Design review of the part built by this model. Coordinates are the model's own, in mm. A direction names the side the tool comes from. Coordinates: 2 decimals unless noted, no trailing zeros. Write each loop counter-clockwise with the first axis right and the second up, starting at its lowest first coordinate (ties: lowest second). Pieces come first, ordered by that corner, then holes. Notation, with made-up numbers: (82, -2.5) - (113, -2.5) arc R8 ccw to (113, 2.5) - close; hole circle Ø2 at (79.5, 23.25). An arc over 180 degrees is marked (long way). One line per item, written item: value.
Autodesk Inventor part; units mm, degrees
ref_plane "YZ Plane" through (0, 0, 0) normal (1, 0, 0) x (0, 1, 0)
ref_plane "XZ Plane" through (0, 0, 0) normal (0, 1, 0) x (-1, 0, 0)
ref_plane "XY Plane" through (0, 0, 0) normal (0, 0, 1) x (1, 0, 0)
sketch "Sketch1" plane through (0, 0, 0) normal (0, 0, 1) x (1, 0, 0)
  line L0 (19.05, -4) -> (-19.05, -4)
  line L1 (-19.05, -4) -> (-19.05, 4)
  line L2 (-19.05, 4) -> (19.05, 4)
  line L3 (19.05, 4) -> (19.05, -4)
  line L4 (19.05, -4) -> (-19.05, 4) construction
  line L5 (-19.05, -4) -> (19.05, 4) construction
  circle A0 centre (11.05, 0) radius 2.25
  circle A1 centre (3.05, 0) radius 2.25
  circle A2 centre (-4.95, 0) radius 2.25
  circle A3 centre (-12.95, 0) radius 2.25
  line L6 (-19.05, 4) -> (-25.4, 4)
  line L7 (-25.4, 4) -> (-25.4, -34.1)
  line L8 (-25.4, -34.1) -> (-19.05, -34.1)
  line L9 (-19.05, -34.1) -> (-19.05, 4)
  line L10 (-25.4, -34.1) -> (-12.6924, -34.1) construction
  line L11 (-25.4, -34.1) -> (-6.35, -34.1)
  line L12 (-6.35, -34.1) -> (-6.35, -27.75)
  line L13 (-6.35, -27.75) -> (-25.4, -27.75)
  line L14 (-25.4, -27.75) -> (-25.4, -34.1)
  line L15 (-6.35, -34.1) -> (-17.257, -23.193)
  point P0 (0, 0)
  point P1 (-19.05, -27.75)
  point P2 (-12.7, -27.75)
  point P3 (-19.05, -27.75)
  dimension "d0" = 38.1
  dimension "d1" = 8
  dimension "d2" = 4.5
  dimension "d3" = 8
  dimension "d4" = 4.5
  dimension "d5" = 8
  dimension "d6" = 4.5
  dimension "d7" = 8
  dimension "d8" = 4.5
  dimension "d9" = 8
  dimension "d10" = 4
  dimension "d11" = 4
  dimension "d12" = 4
  dimension "d13" = 4
  dimension "d16" = 6.35
  dimension "d17" = 38.1
  dimension "d20" = 19.05
  dimension "d21" = 6.35
  dimension "d22" = 45
extrude "Extrusion1" add sketch "Sketch1" along normal blind 6.35 contours L0 L1 L2 L3 | L9 L13 L7 L6 L1 | L13 L15 L11 L9 | L9 L8 L7 L13
fillet "Fillet1" radius 3.175 5 edges at (-19.05, -27.75, 3.175) (-19.05, -4, 3.175) (-25.4, 4, 3.175) (19.05, 4, 3.175) (19.05, -4, 3.175)
fillet "Fillet2" radius 3.175 2 edges at (-12.7, -27.75, 3.175) (-25.4, -34.1, 3.175)
properties part number "CS_Latch_Hooks"
1. For faces 1 (the face through (-3, 4, 3)), 2 (the face through (-15, -27.75, 3)), list the 3-axis set-ups (+Z, -Z, +X, -X, +Y, -Y) from which the entire face can be reached by the end or side of a thin tool; tool diameter is ignored.
Answer block:
face 1: +Z, -Z, +X, -X, +Y
face 2: +Z, -Z, +X
2. Consider section B-B, the plane z = 1. Write out the cut boundary in (x, y) (3 decimals).
Answer block:
outline: (-25.4, -30.925) arc R3.175 ccw to (-22.225, -34.1) - (-6.35, -34.1) - (-11.77, -28.68) arc R3.175 ccw to (-14.015, -27.75) - (-15.875, -27.75) arc R3.175 cw to (-19.05, -24.575) - (-19.05, -7.175) arc R3.175 cw to (-15.875, -4) - (15.875, -4) arc R3.175 ccw to (19.05, -0.825) - (19.05, 0.825) arc R3.175 ccw to (15.875, 4) - (-22.225, 4) arc R3.175 ccw to (-25.4, 0.825) - close; hole circle Ø4.5 at (-12.95, 0); hole circle Ø4.5 at (-4.95, 0); hole circle Ø4.5 at (3.05, 0); hole circle Ø4.5 at (11.05, 0)
3. Mouldability with a two-part tool opening along Y and no side actions: class faces 3 (the face through (-9.9, -3.7, 6.35)), 4 (the face through (18.14, 3.05, 3.22)), 5 (the face through (-7.198, -0.099, 3.131)) as released by +Y, released by -Y, zero draft, split by the parting line, or undercut.
Answer block:
face 3: zero draft
face 4: released by +Y
face 5: undercut
4. Consider section C-C, the plane x = 2. Write out the cut boundary in (y, z), then the cut area to 3 significant figures.
Answer block:
outline: (-4, 0) - (-1.99, 0) - (-1.99, 6.35) - (-4, 6.35) - close; (1.99, 0) - (4, 0) - (4, 6.35) - (1.99, 6.35) - close
area: 25.5 mm^2
5. Wall thickness on line 1 along Y through (x, z) = (-4.95, 2); line 2 along Y through (x, z) = (-12.95, 3); line 3 along Y through (x, z) = (1.5, 1.5): over which ranges is each line inside the solid? List them lowest first.
Answer block:
line 1: y = -4 to -2.25, 2.25 to 4
line 2: y = -34.1 to -27.93, -4 to -2.25, 2.25 to 4
line 3: y = -4 to -1.63, 1.63 to 4
6. Insertion check: pin 1 Ø2.5 at (x, y) = (-4.95, 0) entering from -Z; pin 2 Ø1.5 at (x, z) = (5.5, 1.5) entering from -Y. Each pin has a flat end and moves straight along its axis. Give the tip position at first contact, or say it passes through.
Answer block:
pin 1: passes through
pin 2: stops at y = -4
7. Consider section A-A, the plane y = 0. Write out the cut boundary in (x, z).
Answer block:
outline: (-25.4, 0) - (-15.2, 0) - (-15.2, 6.35) - (-25.4, 6.35) - close; (-10.7, 0) - (-7.2, 0) - (-7.2, 6.35) - (-10.7, 6.35) - close; (-2.7, 0) - (0.8, 0) - (0.8, 6.35) - (-2.7, 6.35) - close; (5.3, 0) - (8.8, 0) - (8.8, 6.35) - (5.3, 6.35) - close; (13.3, 0) - (19.05, 0) - (19.05, 6.35) - (13.3, 6.35) - close
8. Consider section D-D, the plane x = -13. Write out the cut boundary in (y, z).
Answer block:
outline: (-34.1, 0) - (-27.92, 0) - (-27.92, 6.35) - (-34.1, 6.35) - close; (-4, 0) - (-2.25, 0) - (-2.25, 6.35) - (-4, 6.35) - close; (2.25, 0) - (4, 0) - (4, 6.35) - (2.25, 6.35) - close
